from build123d import *

# Parameters (mm, degrees)
F0_R     = 11
F1_DEPTH = 3


with BuildPart() as f1:
    # F0 (on Top) → F1 (new body)
    with BuildSketch(Plane.XY):
        with BuildLine():
            ThreePointArc((12.260471, 6.758762), (11.190713, 8.412368), (9.899495, 9.899495))
            ThreePointArc((9.899495, 9.899495), (8.529441, 11.10174), (7.014803, 12.115797))
            Line((7.014803, 12.115797), (13.47055, 19.752768))
            Line((13.47055, 19.752768), (13.184201, 29.748668))
            Line((13.184201, 29.748668), (6.301852, 37.003547))
            ThreePointArc((6.301852, 37.003547), (0.085743, 36.268282), (-6.148871, 36.825252))
            Line((-6.148871, 36.825252), (-12.820655, 29.376273))
            Line((-12.820655, 29.376273), (-12.820655, 19.376273))
            Line((-12.820655, 19.376273), (-6.758762, 12.260471))
            ThreePointArc((-6.758762, 12.260471), (-8.412368, 11.190713), (-9.899495, 9.899495))
            ThreePointArc((-9.899495, 9.899495), (-11.10174, 8.529441), (-12.115797, 7.014803))
            Line((-12.115797, 7.014803), (-19.752768, 13.47055))
            Line((-19.752768, 13.47055), (-29.748668, 13.184201))
            Line((-29.748668, 13.184201), (-37.003547, 6.301852))
            ThreePointArc((-37.003547, 6.301852), (-36.268282, 0.085743), (-36.825252, -6.148871))
            Line((-36.825252, -6.148871), (-29.376273, -12.820655))
            Line((-29.376273, -12.820655), (-19.376273, -12.820655))
            Line((-19.376273, -12.820655), (-12.260471, -6.758762))
            ThreePointArc((-12.260471, -6.758762), (-11.190713, -8.412368), (-9.899495, -9.899495))
            ThreePointArc((-9.899495, -9.899495), (-8.529441, -11.10174), (-7.014803, -12.115797))
            Line((-7.014803, -12.115797), (-13.47055, -19.752768))
            Line((-13.47055, -19.752768), (-13.184201, -29.748668))
            Line((-13.184201, -29.748668), (-6.301852, -37.003547))
            ThreePointArc((-6.301852, -37.003547), (-0.085743, -36.268282), (6.148871, -36.825252))
            Line((6.148871, -36.825252), (12.820655, -29.376273))
            Line((12.820655, -29.376273), (12.820655, -19.376273))
            Line((12.820655, -19.376273), (6.758762, -12.260471))
            ThreePointArc((6.758762, -12.260471), (8.412368, -11.190713), (9.899495, -9.899495))
            ThreePointArc((9.899495, -9.899495), (11.10174, -8.529441), (12.115797, -7.014803))
            Line((12.115797, -7.014803), (19.752768, -13.47055))
            Line((19.752768, -13.47055), (29.748668, -13.184201))
            Line((29.748668, -13.184201), (37.003547, -6.301852))
            ThreePointArc((37.003547, -6.301852), (36.268282, -0.085743), (36.825252, 6.148871))
            Line((36.825252, 6.148871), (29.376273, 12.820655))
            Line((29.376273, 12.820655), (19.376273, 12.820655))
            Line((19.376273, 12.820655), (12.260471, 6.758762))
        make_face()
        with Locations((-0.256042, -24.376267)):
            Circle(F0_R, mode=Mode.SUBTRACT)
        with Locations((24.376267, -0.256042)):
            Circle(F0_R, mode=Mode.SUBTRACT)
        with Locations((-24.376267, 0.256042)):
            Circle(F0_R, mode=Mode.SUBTRACT)
        with BuildLine():
            ThreePointArc((-7.778175, 7.778175), (0, 11), (7.778175, 7.778175))
            ThreePointArc((7.778175, 7.778175), (11, 0), (7.778175, -7.778175))
            ThreePointArc((7.778175, -7.778175), (0, -11), (-7.778175, -7.778175))
            ThreePointArc((-7.778175, -7.778175), (-11, 0), (-7.778175, 7.778175))
        make_face(mode=Mode.SUBTRACT)
        with Locations((0.256042, 24.376267)):
            Circle(F0_R, mode=Mode.SUBTRACT)
    extrude(amount=F1_DEPTH)


solid = f1.part
Geometry: final body of the model. Coordinates: model frame, mm. A direction names the side the tool comes from. Coordinates: 2 decimals unless noted, no trailing zeros. Loops run counter-clockwise (first coordinate to the right, second up) from the corner with the lowest first, then second, coordinate; pieces in that order, holes last. Notation, with made-up numbers: (30, 49.25) - (88, 49.25) arc R20 cw to (88, 71.25) - close; hole circle Ø3 at (86, 45.5). An arc over 180 degrees is marked (long way). One line per question, with ' | ' between items. Start each with the question number.
(1) Cut plane D-D on y = 3.5. Output: boundary loops of the cut face in (x, z).
(2) Reachability of faces 5 (the flat face through (12.821, -24, 1)), 6 (the flat face through (-12.821, 24, 1)), 7 (the cylindrical face through (36.27, -0.17, 1.48)) from +Z, -Z, +X, -X, +Y, -Y: full face, straight path, thin tool, end or side. Return the list, or none.
(3) Cut plane B-B on y = 28. Output: boundary loops of the cut face in (x, z), and give its area (3 significant figures).
(4) Ray query, L1, parallel to Y at x = -6.5, z = 0.3; L2, parallel to Y at x = 9, z = 2.45; L3, parallel to X at y = 34.5, z = 0.75. Return the intervals inside material, ascending. Write a range as from..to.
(5) Cut plane C-C on x = 5. Output: boundary loops of the cut face in (y, z), and give its area (3 significant figures).
(6) Draft query along Y for faces 1 (the flat face through (24, 12.821, 1)), 2 (the cylindrical face through (-8.55, -11.086, 1.479)), 3 (the flat face through (3, -11, 0)), 4 (the cylindrical face through (-0.17, -36.27, 1.48)). Return one class per face: +Y half, -Y half, draft (parallel to the pull), parting line (faces both ways), or undercut.
(7) Cut plane A-A on x = 15.5. Output: boundary loops of the cut face in (y, z).
(8) First-contact query: pin 1 (1.5 mm diameter, centred on y = -19.5, z = 1, fed in from +X); pin 2 (0.9 mm diameter, centred on y = 22, z = 2, fed in from -X); pin 3 (1.5 mm diameter, centred on x = -22.5, z = 1.5, fed in from -Y). Flat tips, straight axial feed; report the tip coordinate or a pass-through.
Here are the results:
1) outline: (-36.51, 0) - (-34.89, 0) - (-34.89, 3) - (-36.51, 3) - close; (-13.87, 0) - (-10.43, 0) - (-10.43, 3) - (-13.87, 3) - close; (10.43, 0) - (14.04, 0) - (14.04, 3) - (10.43, 3) - close; (34.72, 0) - (36.43, 0) - (36.43, 3) - (34.72, 3) - close
2) face 5: +Z, -Z, +X, -Y | face 6: +Z, -Z, -X, +Y | face 7: +Z, -Z, +X
3) outline: (-12.82, 0) - (-10.13, 0) - (-10.13, 3) - (-12.82, 3) - close; (10.64, 0) - (13.23, 0) - (13.23, 3) - (10.64, 3) - close | area: 15.8 mm²
4) L1: -36.79..-33.43, -15.32..-8.87, 8.87..15.7, 33.06..36.43 | L2: -33.64..-30.32, -18.43..-14.89, -10.72..-6.32, 6.32..10.72, 14.46..17.7, 31.05..34.16 | L3: -8.23..-4.05, 4.56..8.68
5) outline: (-36.62, 0) - (-34.04, 0) - (-34.04, 3) - (-36.62, 3) - close; (-14.71, 0) - (-9.8, 0) - (-9.8, 3) - (-14.71, 3) - close; (9.8, 0) - (14.45, 0) - (14.45, 3) - (9.8, 3) - close; (34.3, 0) - (36.74, 0) - (36.74, 3) - (34.3, 3) - close | area: 43.8 mm²
6) face 1: +Y half | face 2: undercut | face 3: draft | face 4: -Y half
7) outline: (-9.88, 0) - (-6.75, 0) - (-6.75, 3) - (-9.88, 3) - close; (6.24, 0) - (9.52, 0) - (9.52, 3) - (6.24, 3) - close
8) pin 1: x = 12.82 | pin 2: x = -12.82 | pin 3: y = -12.82
